Geometry check sheet. Reference: the model listing, model coordinates, mm. A direction names the side the tool comes from. Coordinates: 2 decimals unless noted, no trailing zeros. Loops run counter-clockwise (first coordinate to the right, second up) from the corner with the lowest first, then second, coordinate; pieces in that order, holes last. Notation, with made-up numbers: (25, 74.5) - (46, 74.5) arc R30 ccw to (46, 107.5) - close; hole circle Ø1 at (60, -31). An arc over 180 degrees is marked (long way). One line per item, written item: value.
from build123d import *

# Parameters (mm, degrees)
F0_W     = 38.1
F0_H     = 38.1
F1_DEPTH = 38.1
F5_DEPTH = 38.1


with BuildPart() as f1:
    # F0 (on Front) → F1 (new body)
    with BuildSketch(Plane.XZ):
        with Locations((19.05, 19.05)):
            Rectangle(F0_W, F0_H)
    extrude(amount=F1_DEPTH)

    # F4 (on offset) → F5 (cut)
    with BuildSketch(Plane.YZ.offset(38.1)):
        Polygon((-11.43, 15.875), (-6.35, 38.1), (-31.75, 38.1), (-26.67, 15.875), (-20.874323, 28.575), (-15.794323, 28.575), align=None)
        Polygon((-31.75, 0), (-38.1, 38.1), (-38.1, 0), align=None)
        Polygon((-25.4, 0), (-12.7, 0), (-19.05, 15.875), align=None)
        Polygon((-6.35, 0), (0, 0), (0, 38.1), align=None)
    extrude(amount=-F5_DEPTH, mode=Mode.SUBTRACT)


solid = f1.part
(1) Cross-section at D-D on y = -3. Record the cut outline in (x, z).
Reply:
outline: (0, 20.1) - (38.1, 20.1) - (38.1, 38.1) - (0, 38.1) - close
(2) Access from +Z, -Z, +X, -X, +Y, -Y to the whole of each face (thin tool, end or side, straight path). Record for faces 5 (the face through (19.32, -15.83, 7.83)), 6 (the face through (19.32, -13.64, 22.31)), 7 (the face through (19, -29, 0)).
Reply:
face 5: -Z, +X, -X
face 6: +Z, +X, -X
face 7: -Z, +X, -X, +Y, -Y
(3) Release check for a two-part mould opening along Y. For faces 1 (the face through (19, -18, 28.575)), 2 (the face through (19, -35, 38.1)), 3 (the face through (19.32, -34.88, 18.78)), 4 (the face through (19.3, -22.2, 8)) record: pulls with the +Y half, pulls with the -Y half, needs draft (parallel to the pull), parting line crosses it, or undercut.
Reply:
face 1: undercut
face 2: needs draft
face 3: pulls with the -Y half
face 4: undercut
(4) Go/stop test with flat-tipped pins: pin 1 Ø8 at (x, z) = (10.5, 19) entering from -Y; pin 2 Ø10 at (x, z) = (15.5, 29) entering from +Y; pin 3 Ø2.5 at (x, y) = (19, -18.5) entering from +Z (3 decimals). Record where each tip stops, or that it passes through.
Reply:
pin 1: y = -35.58
pin 2: y = -0.68
pin 3: z = 28.575
(5) Cross-section at A-A on z = 29.5. Record the cut outline in (x, y).
Reply:
outline: (0, -36.67) - (38.1, -36.67) - (38.1, -29.78) - (0, -29.78) - close; (0, -8.32) - (38.1, -8.32) - (38.1, -1.43) - (0, -1.43) - close
(6) Cross-section at B-B on x = 28.5. Record the cut outline in (y, z) (3 decimals), and give its area (3 significant figures).
Reply:
outline: (-38.1, 38.1) - (-31.75, 0) - (-25.4, 0) - (-19.05, 15.875) - (-12.7, 0) - (-6.35, 0) - (0, 38.1) - (-6.35, 38.1) - (-11.43, 15.875) - (-15.794, 28.575) - (-20.874, 28.575) - (-26.67, 15.875) - (-31.75, 38.1) - close
area: 786 mm2
(7) Material ranges on probe 1 along Y at (x, z) = (15.5, 17.5); probe 2 along Y at (x, z) = (10.5, 27); probe 3 along Y at (x, z) = (18, 3), recorded low to high. Write a range as from..to.
Reply:
probe 1: -34.67..-27.04, -25.93..-11.99, -11.06..-3.43
probe 2: -36.25..-29.21, -21.59..-15.25, -8.89..-1.85
probe 3: -32.25..-24.2, -13.9..-5.85
(8) Cross-section at C-C on z = 20.5. Record the cut outline in (x, y).
Reply:
outline: (0, -35.17) - (38.1, -35.17) - (38.1, -27.73) - (0, -27.73) - close; (0, -24.56) - (38.1, -24.56) - (38.1, -13.02) - (0, -13.02) - close; (0, -10.37) - (38.1, -10.37) - (38.1, -2.93) - (0, -2.93) - close
